Read the model definition and answer for the solid it produces. Units are mm, in the model's axes. A direction names the side the tool comes from. Round coordinates to 2 decimals unless told otherwise and drop trailing zeros. Order: outer loops, then holes, each group sorted by start corner. A loop starts at its lowest first (then second) coordinate and runs counter-clockwise, first axis right, second up. Notation, with made-up numbers: (34.25, 72) - (80.25, 72) arc R24 ccw to (80.25, 96) - close; hole circle Ø8 at (-9.75, 88). An arc over 180 degrees is marked (long way). One line per question, with ' | ' between items. Start each with the question number.
1) The mould has two halves that part along Y. Classify faces 3 (the cylindrical face through (29.36, 5.37, 1.19)), 4 (the flat face through (55, 0, 3)), 5 (the cylindrical face through (48.92, -2.44, -0.54)): pulls with the +Y half, pulls with the -Y half, needs draft (parallel to the pull), parting line crosses it, or undercut.
2) The part is cut by section C-C, the plane z = -6.25. Give the vertices of the cut face in (x, y).
3) For faces 1 (the flat face through (3, 5, -3)), 2 (the flat face through (0, 0, 0)), determine the directions among +Z, -Z, +X, -X, +Y, -Y from which every point of the face is accessible in a straight line to the end or side of a thin tool.
4) The part is cut by section B-B, the plane x = 14. Give the vertices of the cut face in (y, z).
5) Straight lines are drawn through the part: line 1 (Y direction, x = 48, z = 0); line 2 (X direction, y = -6, z = 2.75); line 3 (Y direction, x = 48, z = 2). For each, find the intervals that lie inside material, in ascending order. Write a range as from..to.
6) Flat-ended cylindrical pins translate along their axes: pin 1 (2 mm diameter, centred on x = 7.5, z = -2, fed in from -Y); pin 2 (1.5 mm diameter, centred on x = 44.5, y = -2, fed in from +Z); pin 3 (3 mm diameter, centred on x = 19, z = 4.5, fed in from -Y); pin 4 (6 mm diameter, centred on y = 0, z = 0, fed in from -X). Find the tip coordinate at first contact, or state that the pin passes through.
7) The part is cut by section A-A, the plane z = 3. Give the vertices of the cut face in (x, y), plus the area to 3 significant figures.
from build123d import *

# Parameters (mm, degrees)
BROCA_DE_ROSQUEAR_PARA_TARRAXA_DE_M61_D     = 5
BROCA_DE_ROSQUEAR_PARA_TARRAXA_DE_M61_DEPTH = 12
BROCA_DE_ROSQUEAR_PARA_TARRAXA_DE_M61_TIP   = 1.502151548


with BuildPart() as part:
    # Sketch1 → Revolve1 (revolve)
    with BuildSketch(Plane.XY, mode=Mode.PRIVATE) as revolve1_sk:
        Polygon((0, 0), (0, 7.7), (3, 7.7), (3, 5.5), (55, 5.5), (55, 0), align=None)
    revolve(revolve1_sk.sketch.rotate(Axis((0, 0, 0), (-1, 0, 0)), 90), axis=Axis((0, 0, 0), (-1, 0, 0)))

    # Broca de rosquear para tarraxa de M61
    with Locations(Plane(origin=(55, 0, 0), x_dir=(0, 0, -1), z_dir=(1, 0, 0))):
        with Locations((0, 0)):
            Hole(BROCA_DE_ROSQUEAR_PARA_TARRAXA_DE_M61_D / 2, depth=BROCA_DE_ROSQUEAR_PARA_TARRAXA_DE_M61_DEPTH)
            with Locations((0, 0, -(BROCA_DE_ROSQUEAR_PARA_TARRAXA_DE_M61_DEPTH + BROCA_DE_ROSQUEAR_PARA_TARRAXA_DE_M61_TIP / 2))):  # 118° drill point
                Cone(0, BROCA_DE_ROSQUEAR_PARA_TARRAXA_DE_M61_D / 2, BROCA_DE_ROSQUEAR_PARA_TARRAXA_DE_M61_TIP, mode=Mode.SUBTRACT)


solid = part.part
Values:
1) face 3: parting line crosses it | face 4: needs draft | face 5: undercut
2) outline: (0, -4.5) - (3, -4.5) - (3, 4.5) - (0, 4.5) - close
3) face 1: +X | face 2: +Z, -Z, -X, +Y, -Y
4) outline: circle Ø11 at (0, 0)
5) line 1: y = -5.5..-2.5, 2.5..5.5 | line 2: x = 0..3 | line 3: y = -5.12..-1.5, 1.5..5.12
6) pin 1: stops at y = -5.41 | pin 2: stops at z = 5.36 | pin 3: stops at y = -4.61 | pin 4: stops at x = 0
7) outline: (0, -7.09) - (3, -7.09) - (3, -4.61) - (55, -4.61) - (55, 4.61) - (3, 4.61) - (3, 7.09) - (0, 7.09) - close | area: 522 mm^2
